Part model, mm, in its own coordinate system. A direction names the side the tool comes from. Coordinates: 2 decimals unless noted, no trailing zeros. Order: outer loops, then holes, each group sorted by start corner. A loop starts at its lowest first (then second) coordinate and runs counter-clockwise, first axis right, second up.
1) Cut at C-C (y = -177.8). Give the number of separate pieces and of enclosed holes in the cut face, and give its area (3 significant figures).
2) Pin check, flat tips, straight feed: pin 1 Ø14 at (x, y) = (28.5, -176) entering from +Z; pin 2 Ø1.5 at (x, y) = (136.5, -32.5) entering from +Z; pin 3 Ø2 at (y, z) = (-119, 119) entering from +X. Stop position of each tip, or through.
3) Tool access for faces 5 (the cylindrical face through (20.72, -173.51, 23.54)), 6 (the flat face through (25, -178, 34.696)), 7 (the flat face through (101, -190.5, 74)): list every direction of +Z, -Z, +X, -X, +Y, -Y with a clear straight run to the whole face (end or side of a thin tool).
4) Cut at B-B (x = 25.4). List the corners of the cut face in (y, z), and give its area (3 significant figures).
5) Mould opens along Z. For faces 1 (the cylindrical face through (118.185, -37.412, 94.881)), 2 (the flat face through (30, -94, 12.7)), 3 (the flat face through (122.74, -93.92, 89.89)), 4 (the flat face through (0, -94, 6)) say: +Z half, -Z half, draft (parallel to the pull), parting line (faces both ways), or undercut.
6) Cut at A-A (y = -127.5). List the corners of the cut face in (x, z) (1 decimal).
7) Wall check: L1, parallel to Z at x = 58, y = -121; L2, parallel to X at y = -97, z = 12; L3, parallel to Z at x = 63, y = -108. Give the ranges that are in metal, low to high.
8) Cut at D-D (z = 177.5). List the corners of the cut face in (x, y).
```python
from build123d import *

# Parameters (mm, degrees)
F1_DEPTH = 190.5
F2_R     = 3.175
F3_DEPTH = 25.4
F4_R     = 6.35
F5_DEPTH = 10.9982
F6_R     = 6.35
F7_DEPTH = 21.9964


with BuildPart() as f1:
    # F0 (on Front) → F1 (new body)
    with BuildSketch(Plane.XZ):
        with BuildLine():
            Line((0, 12.7), (0, 0))
            Line((0, 0), (70.8406, 0))
            Line((70.8406, 0), (176.1109, 182.333508128))
            Line((176.1109, 182.333508128), (165.1123773719, 188.683508128))
            Line((165.1123773719, 188.683508128), (65.8874360053, 16.820868303))
            ThreePointArc((65.8874360053, 16.820868303), (65.878154986, 8.573768655), (58.7375, 12.7))
            Line((58.7375, 12.7), (0, 12.7))
        make_face()
    extrude(amount=F1_DEPTH)

    # F2 (on face) → F3 (cut)
    with BuildSketch(Plane(origin=(42.1319273719, 0, -24.3248796097), x_dir=(0, -1, 0), z_dir=(-0.8660254038, 0, 0.5))):
        with Locations((38.1, 144.3609)):
            Circle(F2_R)
        with Locations((114.3, 144.3609)):
            Circle(F2_R)
        with Locations((177.8, 144.3609)):
            Circle(F2_R)
        with Locations((177.8, 195.1609)):
            Circle(F2_R)
    extrude(amount=-F3_DEPTH, mode=Mode.SUBTRACT)

    # F4 (on face) → F5 (join)
    with BuildSketch(Plane(origin=(42.1319273719, 0, -24.3248796097), x_dir=(0, -1, 0), z_dir=(-0.8660254038, 0, 0.5))):
        with Locations((177.8, 80.8609)):
            Circle(F4_R)
    extrude(amount=F5_DEPTH)

    # F6 (on face) → F7 (join)
    with BuildSketch(Plane.XY.offset(12.7)):
        with Locations((25.4, -177.8)):
            Circle(F6_R)
    extrude(amount=F7_DEPTH)


solid = f1.part
```
Geometry check:
1. separate pieces: 3
1. enclosed holes: 0
1. area: 3,690 mm2
2. pin 1: stops at z = 34.7
2. pin 2: stops at z = 140.42
2. pin 3: stops at x = 140.12
3. face 5: +Z
3. face 6: +Z, -X, +Y, -Y
3. face 7: +Z, -Z, +X, -X, -Y
4. outline: (-190.5, 0) - (0, 0) - (0, 12.7) - (-171.45, 12.7) - (-171.45, 34.7) - (-184.15, 34.7) - (-184.15, 12.7) - (-190.5, 12.7) - close
4. area: 2,700 mm2
5. face 1: undercut
5. face 2: +Z half
5. face 3: -Z half
5. face 4: draft
6. outline: (0, 0) - (70.8, 0) - (176.1, 182.3) - (165.1, 188.7) - (65.9, 16.8) arc R4.8 cw (long way) to (58.7, 12.7) - (0, 12.7) - close
7. L1: z = 0 to 12.7
7. L2: x = 0 to 58.79, 68.21 to 77.77
7. L3: z = 0 to 7.96
8. outline: (158.66, -190.5) - (173.32, -190.5) - (173.32, 0) - (158.66, 0) - close
